```python
from build123d import *

# Parameters (mm, degrees)
F0_R     = 39.669031
F1_DEPTH = 50.8
F2_W     = 164.8714
F2_H     = 22.5044
F3_DEPTH = 50.8
F4_R     = 29.483295
F5_DEPTH = 25.4


with BuildPart() as f1:
    # F0 (on Top) → F1 (new body)
    with BuildSketch(Plane.XY):
        Circle(F0_R)
    extrude(amount=F1_DEPTH)

    # F2 (on face) → F3 (join)
    with BuildSketch(Plane.XY.offset(50.8)):
        with Locations((43.408703, 4.14407)):
            Rectangle(F2_W, F2_H)
    extrude(amount=F3_DEPTH)

    # F4 (on face) → F5 (join)
    with BuildSketch(Plane.XY.offset(101.6)):
        with Locations((96.361108, 4.14407)):
            Circle(F4_R)
    extrude(amount=F5_DEPTH)


solid = f1.part
```
Input: part model. Units: mm. Frame: model coordinates. A direction names the side the tool comes from. Give positions to 0.01 mm unless a question says otherwise; leave off trailing zeros. Loops run counter-clockwise (first coordinate to the right, second up) from the corner with the lowest first, then second, coordinate; pieces in that order, holes last.
1) Line query: L1, parallel to Y at x = 84, z = 92; L2, parallel to Z at x = -6, y = -3.5; L3, parallel to Z at x = 97, y = -7.5. Output: solid intervals per line, ascending.
A:
L1: y = -7.11 to 15.4
L2: z = 0 to 101.6
L3: z = 101.6 to 127
2) Section query A-A on x = 0. Return the cut outline in (y, z), and give its area (3 significant figures).
A:
outline: (-39.67, 0) - (39.67, 0) - (39.67, 50.8) - (15.4, 50.8) - (15.4, 101.6) - (-7.11, 101.6) - (-7.11, 50.8) - (-39.67, 50.8) - close
area: 5,170 mm2
3) Mould query, pull axis Y, two halves, no side actions, for faces 6 (the cylindrical face through (66.906, 5.44, 114.122)), 7 (the flat face through (42, 15.396, 76)), 8 (the flat face through (-1, 25, 50.8)), 9 (the flat face through (42, -7.108, 76)). Classes: released by +Y, released by -Y, zero draft, split by the parting line, or undercut.
A:
face 6: split by the parting line
face 7: released by +Y
face 8: zero draft
face 9: released by -Y
4) Section query C-C on y = 0. Return the cut outline in (x, z).
A:
outline: (-39.67, 0) - (39.67, 0) - (39.67, 50.8) - (125.84, 50.8) - (125.84, 101.6) - (125.55, 101.6) - (125.55, 127) - (67.17, 127) - (67.17, 101.6) - (-39.03, 101.6) - (-39.03, 50.8) - (-39.67, 50.8) - close
5) Section query B-B on y = -10. Return the cut outline in (x, z), and give its area (3 significant figures).
A:
outline: (-38.39, 0) - (38.39, 0) - (38.39, 50.8) - (-38.39, 50.8) - close; (70.49, 101.6) - (122.23, 101.6) - (122.23, 127) - (70.49, 127) - close
area: 5,210 mm2
6) Section query D-D on z = 21. Return the cut outline in (x, y), and give its area (3 significant figures).
A:
outline: circle Ø79.34 at (0, 0)
area: 4,940 mm2
7) Reachability of faces 1 (the flat face through (-39.027, 4, 76)), 2 (the flat face through (-1, -20, 50.8)), 3 (the flat face through (96, 23, 101.6)), 4 (the flat face through (96, -14, 101.6)), 5 (the flat face through (125.844, 4, 76)) from +Z, -Z, +X, -X, +Y, -Y: full face, straight path, thin tool, end or side. Return the list, or none.
A:
face 1: +Z, -X, +Y, -Y
face 2: +Z, +X, -X, -Y
face 3: -Z, +X, -X, +Y
face 4: -Z, +X, -X, -Y
face 5: +Z, -Z, +X, +Y, -Y
8) Contact query for flat-ended pins moving along their axis: pin 1 (18 mm diameter, centred on y = 8.5, z = 68, fed in from -X); pin 2 (15 mm diameter, centred on x = 49, z = 85.5, fed in from +Y); pin 3 (5.5 mm diameter, centred on x = 90.5, y = -19.5, fed in from -Z). Output: stop coordinate, or through.
A:
pin 1: stops at x = -39.03
pin 2: stops at y = 15.4
pin 3: stops at z = 101.6
